For this review, take the finished solid that the model builds, in its own axes (mm). A direction names the side the tool comes from. Round coordinates to 2 decimals unless told otherwise and drop trailing zeros. Write each loop counter-clockwise with the first axis right and the second up, starting at its lowest first coordinate (ties: lowest second). Pieces come first, ordered by that corner, then holes. Notation, with made-up numbers: (-40, 1.25) -> (-36, 1.25) arc R12 cw to (-36, 24.25) -> close; hole circle Ø8 at (56, 13.25). An arc over 180 degrees is marked (long way). Answer in a Markdown table with one row per item.
from build123d import *

# Parameters (mm, degrees)
BOSS_EXTRUDE1_DEPTH             = 2.3876
BOSS_EXTRUDE2_REACH             = 126.668
SKETCH2_W                       = 2.3876
SKETCH2_H                       = 2.3876
BOSS_EXTRUDE2_DIRECTION_2_REACH = 126.668


with BuildPart() as part:
    # Sketch1 → Boss-Extrude1 (new body)
    with BuildSketch(Plane.XY):
        with BuildLine():
            Line((0, 4.91087), (119.637, 4.91087))
            ThreePointArc((119.637, 4.91087), (124.54787, 0), (119.637, -4.91087))
            Line((119.637, -4.91087), (0, -4.91087))
            ThreePointArc((0, -4.91087), (-4.91087, 0), (0, 4.91087))
        make_face()
        with BuildLine():
            Line((0, 3.25), (119.637, 3.25))
            ThreePointArc((119.637, 3.25), (122.887, 0), (119.637, -3.25))
            Line((119.637, -3.25), (0, -3.25))
            ThreePointArc((0, -3.25), (-3.25, 0), (0, 3.25))
        make_face(mode=Mode.SUBTRACT)
    extrude(amount=-BOSS_EXTRUDE1_DEPTH)

    # Sketch2 → Boss-Extrude2 (add, up to next)
    with BuildSketch(Plane(origin=(0, 0, 0), x_dir=(1, 0, 0), z_dir=(0, 1, 0)), mode=Mode.PRIVATE) as boss_extrude2_sk1:
        with Locations((59.8185, 1.1938)):
            Rectangle(SKETCH2_W, SKETCH2_H)
    boss_extrude2_tool1 = extrude(boss_extrude2_sk1.sketch, amount=BOSS_EXTRUDE2_REACH, mode=Mode.PRIVATE) - part.part
    add(boss_extrude2_tool1.solids().sort_by_distance((59.8185, 0, -1.1938))[0])

    # Sketch2 → Boss-Extrude2 direction 2 (add, up to next)
    with BuildSketch(Plane(origin=(0, 0, 0), x_dir=(1, 0, 0), z_dir=(0, 1, 0)), mode=Mode.PRIVATE) as boss_extrude2_direction_2_sk1:
        with Locations((59.8185, 1.1938)):
            Rectangle(SKETCH2_W, SKETCH2_H)
    boss_extrude2_direction_2_tool1 = extrude(boss_extrude2_direction_2_sk1.sketch, amount=-BOSS_EXTRUDE2_DIRECTION_2_REACH, mode=Mode.PRIVATE) - part.part
    add(boss_extrude2_direction_2_tool1.solids().sort_by_distance((59.8185, 0, -1.1938))[0])


solid = part.part
1) Clearance check with flat-ended pins moving along their axes: pin 1 Ø0.7 at (y, z) = (1, -1) entering from -X; pin 2 Ø1 at (y, z) = (3.5, -1) entering from +X (3 decimals). State where each tip first meets the part, or that it passes through.
Solved:
| item | result |
|---|---|
| pin 1 | x = -4.87 |
| pin 2 | x = 123.525 |
2) Consider section C-C on z = -1.75. State the section outline as (x, y) points.
Solved:
| item | result |
|---|---|
| outline | (0, -4.91) -> (119.64, -4.91) arc R4.91 ccw to (119.64, 4.91) -> (0, 4.91) arc R4.91 ccw to start; hole (0, -3.25) -> (58.62, -3.25) -> (58.62, 3.25) -> (0, 3.25) arc R3.25 ccw to start; hole (61.01, -3.25) -> (119.64, -3.25) arc R3.25 ccw to (119.64, 3.25) -> (61.01, 3.25) -> close |
3) Consider section A-A on y = 0. State the section outline as (x, z) points.
Solved:
| item | result |
|---|---|
| outline | (-4.91, -2.39) -> (-3.25, -2.39) -> (-3.25, 0) -> (-4.91, 0) -> close; (58.62, -2.39) -> (61.01, -2.39) -> (61.01, 0) -> (58.62, 0) -> close; (122.89, -2.39) -> (124.55, -2.39) -> (124.55, 0) -> (122.89, 0) -> close |
4) Consider section B-B on x = 115. State the section outline as (y, z) points, then the cut area to 3 significant figures.
Solved:
| item | result |
|---|---|
| outline | (-4.91, -2.39) -> (-3.25, -2.39) -> (-3.25, 0) -> (-4.91, 0) -> close; (3.25, -2.39) -> (4.91, -2.39) -> (4.91, 0) -> (3.25, 0) -> close |
| area | 7.93 mm² |
5) For line 1 (X direction, y = -0.25, z = -1.25); line 2 (Y direction, x = 34.5, z = -0.6); line 3 (X direction, y = -2, z = -1.9), list the stretches that pass through material, from the lowest coordinate up. Write a range as [from, to].
Solved:
| item | result |
|---|---|
| line 1 | [-4.9, -3.24], [58.62, 61.01], [122.88, 124.54] |
| line 2 | [-4.91, -3.25], [3.25, 4.91] |
| line 3 | [-4.49, -2.56], [58.62, 61.01], [122.2, 124.12] |
6) For faces 1 (the flat face through (61, -4.911, -1)), 2 (the flat face through (91, -3.25, -1)), list the 3-axis set-ups (+Z, -Z, +X, -X, +Y, -Y) from which the entire face can be reached by the end or side of a thin tool; tool diameter is ignored.
Solved:
| item | result |
|---|---|
| face 1 | +Z, -Z, +X, -X, -Y |
| face 2 | +Z, -Z |
7) Mouldability with a two-part tool opening along X and no side actions: class faces 3 (the flat face through (59, 1, -2.388)), 4 (the cylindrical face through (122.886, 0.071, -1.177)), 5 (the cylindrical face through (-4.91, -0.11, -1.18)), 6 (the flat face through (61.012, 0, -1)) as pulls with the +X half, pulls with the -X half, needs draft (parallel to the pull), parting line crosses it, or undercut.
Solved:
| item | result |
|---|---|
| face 3 | needs draft |
| face 4 | undercut |
| face 5 | pulls with the -X half |
| face 6 | undercut |
